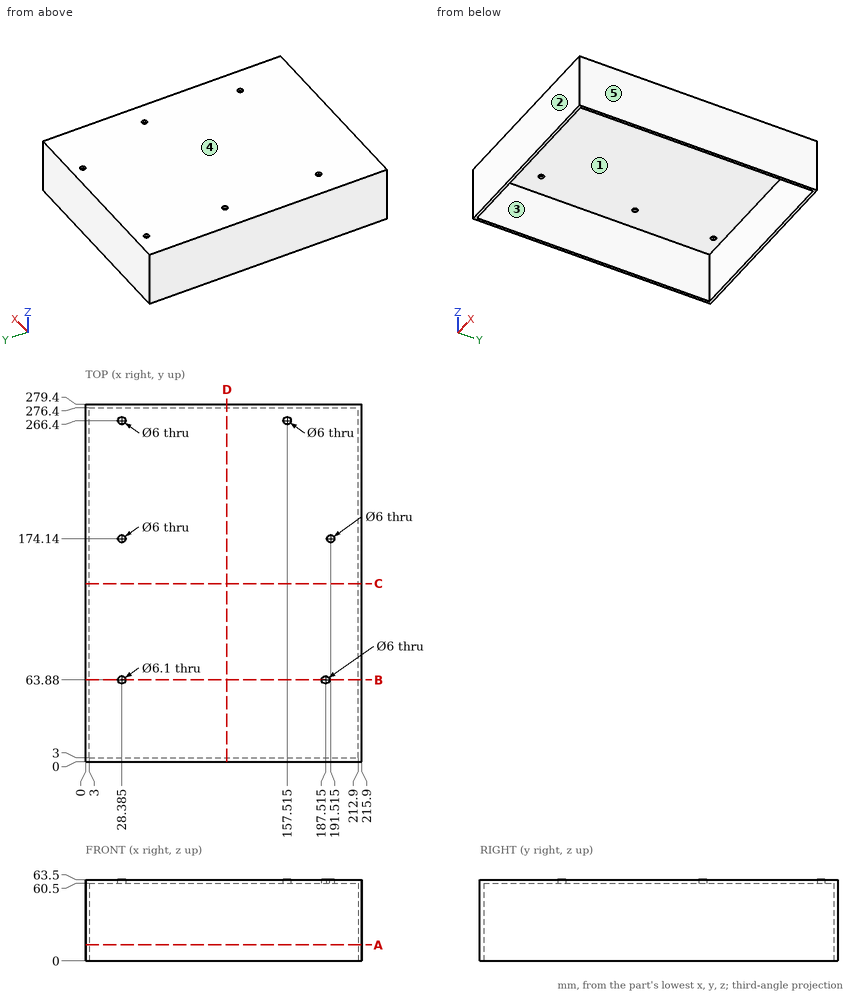
Part print with two shaded views. Sizes in mm from the minimum x, y, z corner. A direction names the side the tool comes from. Round coordinates to 2 decimals unless told otherwise and drop trailing zeros. Loops run counter-clockwise (first coordinate to the right, second up) from the corner with the lowest first, then second, coordinate; pieces in that order, holes last.
Item 1: Saw through at B-B (y = 63.88). List the corners of the cut face in (x, z) (3 decimals).
Item 2: Which spindle directions (+Z, -Z, +X, -X, +Y, -Y) get a long thin tool onto all of the face, cutting with end or side? Do the marked faces 1 and 2. Say none if no direction does.
Item 3: Pin check, flat tips, straight feed: P1, Ø10, axis at x = 153.5, y = 227, coming from the -Z side; P2, Ø3.5, axis at x = 28.385, y = 266.4, coming from the +Z side. Stop position of each tip, or through.
Item 4: Drill centre lines: line 1 along X through (y, z) = (266, 62); line 2 along X through (y, z) = (174.14, 61.2) (3 decimals); line 3 along Y through (x, z) = (104, 59). Where is each one in solid material? Low to high.
Item 5: Saw through at A-A (z = 12.5). List the corners of the cut face in (x, y).
Item 6: Saw through at C-C (y = 139). List the corners of the cut face in (x, z), then the cut area to 3 significant figures.
Item 7: Saw through at D-D (x = 110.5). List the corners of the cut face in (y, z).
Item 8: Two-plate mould, pull along X, no slides. Class the marked faces 3, 4 and 5: released by +X, released by -X, zero draft, split by the parting line, or undercut.
Worked answers:
1. outline: (0, 0) - (3, 0) - (3, 60.5) - (25.335, 60.5) - (25.335, 63.5) - (0, 63.5) - close; (31.435, 60.5) - (184.515, 60.5) - (184.515, 63.5) - (31.435, 63.5) - close; (190.515, 60.5) - (212.9, 60.5) - (212.9, 0) - (215.9, 0) - (215.9, 63.5) - (190.515, 63.5) - close
2. face 1: -Z
2. face 2: +Z, -Z, +X, -X, -Y
3. P1: stops at z = 60.5
3. P2: passes through
4. line 1: x = 0 to 25.41, 31.36 to 154.54, 160.49 to 215.9
4. line 2: x = 0 to 25.385, 31.385 to 188.515, 194.515 to 215.9
4. line 3: y = 0 to 3, 276.4 to 279.4
5. outline: (0, 0) - (215.9, 0) - (215.9, 279.4) - (0, 279.4) - close; hole (3, 3) - (212.9, 3) - (212.9, 276.4) - (3, 276.4) - close
6. outline: (0, 0) - (3, 0) - (3, 60.5) - (212.9, 60.5) - (212.9, 0) - (215.9, 0) - (215.9, 63.5) - (0, 63.5) - close
6. area: 1,010 mm2
7. outline: (0, 0) - (3, 0) - (3, 60.5) - (276.4, 60.5) - (276.4, 0) - (279.4, 0) - (279.4, 63.5) - (0, 63.5) - close
8. face 3: undercut
8. face 4: zero draft
8. face 5: released by +X
